```python
from build123d import *

# Parameters (mm, degrees)
SKETCH_W        = 60
SKETCH_H        = 87
SKETCH_W_2      = 20
SKETCH_H_2      = 52
PAD_DEPTH       = 3
SKETCH001_W     = 60
SKETCH001_H     = 87
SKETCH001_R     = 1.5
SKETCH001_W_2   = 52
SKETCH001_H_2   = 79
PAD001_DEPTH    = 40
SKETCH002_W     = 55
SKETCH002_H     = 47
POCKET_DEPTH    = 3
POCKET001_DEPTH = 4


with BuildPart() as part:
    # Sketch → Pad (new body)
    with BuildSketch(Plane.XY):
        with Locations((30, 43.5)):
            Rectangle(SKETCH_W, SKETCH_H)
        with Locations((20, 51)):
            Rectangle(SKETCH_W_2, SKETCH_H_2, mode=Mode.SUBTRACT)
    extrude(amount=PAD_DEPTH)

    # Sketch001 (on Pad) → Pad001 (join)
    with BuildSketch(Plane.XY):
        with Locations((30, 43.5)):
            Rectangle(SKETCH001_W, SKETCH001_H)
        with Locations((2, 2)):
            Circle(SKETCH001_R, mode=Mode.SUBTRACT)
        with Locations((58, 2)):
            Circle(SKETCH001_R, mode=Mode.SUBTRACT)
        with Locations((2, 85)):
            Circle(SKETCH001_R, mode=Mode.SUBTRACT)
        with Locations((58, 85)):
            Circle(SKETCH001_R, mode=Mode.SUBTRACT)
        with Locations((30, 43.5)):
            Rectangle(SKETCH001_W_2, SKETCH001_H_2, mode=Mode.SUBTRACT)
    extrude(amount=PAD001_DEPTH)

    # Sketch002 (on Face20 of Pad001) → Pocket (cut)
    with BuildSketch(Plane.XY.offset(40)):
        with Locations((30, 61)):
            Rectangle(SKETCH002_W, SKETCH002_H)
    extrude(amount=-POCKET_DEPTH, mode=Mode.SUBTRACT)

    # Sketch003 (on Face26 of Pocket) → Pocket001 (cut)
    with BuildSketch(Plane.YZ.offset(60)):
        with BuildLine():
            ThreePointArc((72.724212, 19.885724), (76.374689, 23.536201), (72.724212, 27.186677))
            Line((72.724212, 27.186677), (51.825985, 27.186677))
            ThreePointArc((51.825985, 27.186677), (48.175508, 23.536201), (51.825985, 19.885724))
            Line((72.724212, 19.885724), (51.825985, 19.885724))
        make_face()
    extrude(amount=-POCKET001_DEPTH, mode=Mode.SUBTRACT)


solid = part.part
```
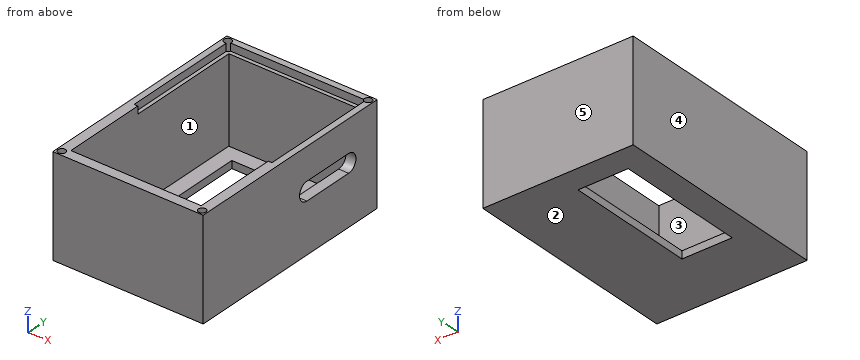
Build history of the part. All positions in model axes, mm. Face numbers are marked on the shaded views. A direction names the side the tool comes from. Round coordinates to 2 decimals unless told otherwise and drop trailing zeros. Write each loop counter-clockwise with the first axis right and the second up, starting at its lowest first coordinate (ties: lowest second). Pieces come first, ordered by that corner, then holes.
1) Band-saw the part on A-A, the plane z = 30.5. List the corners of the cut face in (x, y).
2) Band-saw the part on D-D, the plane y = 75. List the corners of the cut face in (x, z).
3) Band-saw the part on C-C, the plane y = 2. List the corners of the cut face in (x, z), and give its area (3 significant figures).
4) Drill centre lines: probe 1 along Y at (x, z) = (58, 30); probe 2 along X at (y, z) = (85, 19); probe 3 along X at (y, z) = (39, 31). Where is each one in solid material? Low to high.
5) Band-saw the part on B-B, the plane x = 25. List the corners of the cut face in (y, z).
6) Pin check, flat tips, straight feed: pin 1 (10 mm diameter, centred on x = 46, z = 12.5, fed in from -Y); pin 2 (14 mm diameter, centred on x = 28.5, y = 67, fed in from +Z). Stop position of each tip, or through.
7) Mould opens along X. For the marked faces 3, 4 and 5 say: +X half, -X half, draft (parallel to the pull), parting line (faces both ways), or undercut.
8) 3-axis set-ups, long thin cutter, end or side, ignore diameter. For the marked faces 1 and 2: which of +Z, -Z, +X, -X, +Y, -Y reach the whole face in a straight line?
Ans:
1. outline: (0, 0) - (60, 0) - (60, 87) - (0, 87) - close; hole circle Ø3 at (2, 2); hole circle Ø3 at (2, 85); hole (4, 4) - (56, 4) - (56, 83) - (4, 83) - close; hole circle Ø3 at (58, 2); hole circle Ø3 at (58, 85)
2. outline: (0, 0) - (10, 0) - (10, 3) - (4, 3) - (4, 37) - (2.5, 37) - (2.5, 40) - (0, 40) - close; (30, 0) - (60, 0) - (60, 20.68) - (56, 20.68) - (56, 3) - (30, 3) - close; (56, 26.39) - (60, 26.39) - (60, 40) - (57.5, 40) - (57.5, 37) - (56, 37) - close
3. outline: (0, 0) - (60, 0) - (60, 40) - (59.5, 40) - (59.5, 3) - (56.5, 3) - (56.5, 40) - (3.5, 40) - (3.5, 3) - (0.5, 3) - (0.5, 40) - (0, 40) - close
3. area: 2,180 mm2
4. probe 1: y = 0 to 0.5, 3.5 to 83.5, 86.5 to 87
4. probe 2: x = 0 to 0.5, 3.5 to 56.5, 59.5 to 60
4. probe 3: x = 0 to 4, 56 to 60
5. outline: (0, 0) - (25, 0) - (25, 3) - (4, 3) - (4, 40) - (0, 40) - close; (77, 0) - (87, 0) - (87, 40) - (84.5, 40) - (84.5, 37) - (83, 37) - (83, 3) - (77, 3) - close
6. pin 1: stops at y = 0
6. pin 2: stops at z = 3
7. face 3: undercut
7. face 4: -X half
7. face 5: draft
8. face 1: +Z
8. face 2: -Z, +X, -X, +Y, -Y
